Read the model definition and answer for the solid it produces. Units are mm, in the model's axes. Give positions to 0.01 mm unless a question says otherwise; leave off trailing zeros. Order: outer loops, then holes, each group sorted by start corner. A loop starts at its lowest first (then second) coordinate and runs counter-clockwise, first axis right, second up. Notation, with made-up numbers: (-5, 53) - (39, 53) arc R12 cw to (39, 59) - close; hole circle Ø6 at (17.25, -33.75). An arc over 180 degrees is marked (long way). Write each question's results on one line, items separated by ' | '. Start each with the question number.
Q1. Find the intervals of material crossed by line 1 along Z through (x, y) = (-101.5, 1); line 2 along Z through (x, y) = (92.5, 2.85); line 3 along Z through (x, y) = (72, 1.65), in increasing order. Write a range as from..to.
Q2. A flat-ended cylindrical pin translates along its axis: P1, Ø1, axis at y = 2.5, z = -94, coming from the +X side. Find the tip coordinate at first contact, or state that the pin passes through.
Q3. Find section A-A on x = 40. Give the vertices of the cut face in (y, z) (3 decimals), and give its area (3 significant figures).
Q4. Find section B-B on z = -66. Give the vertices of the cut face in (x, y) (3 decimals), and give its area (3 significant figures).
Q5. Find section C-C on y = 1.45. Count the separate pieces of the cut face and the enclosed holes in it, and give its area (3 significant figures).
Autodesk Inventor part; units mm, degrees
ref_plane "YZ Plane" through (0, 0, 0) normal (1, 0, 0) x (0, 1, 0)
ref_plane "XZ Plane" through (0, 0, 0) normal (0, 1, 0) x (-1, 0, 0)
ref_plane "XY Plane" through (0, 0, 0) normal (0, 0, 1) x (1, 0, 0)
sketch "Sketch1" plane through (0, 0, 0) normal (0, 1, 0) x (-1, 0, 0)
  line L0 (147.066, 381) -> (0, 381)
  line L1 (-147.066, 33.688) -> (-147.066, -381)
  line L2 (-147.066, -381) -> (147.066, -381)
  line L3 (147.066, -381) -> (147.066, 381)
  line L4 (147.066, 381) -> (-147.066, -381) construction
  line L5 (136.271, -185.928) -> (115.951, -185.928) construction
  line L6 (115.951, -185.928) -> (115.951, -231.648) construction
  line L7 (115.951, -231.648) -> (136.271, -231.648) construction
  line L8 (136.271, -231.648) -> (136.271, -185.928) construction
  line L9 (136.271, -185.928) -> (115.951, -231.648) construction
  line L10 (115.951, -185.928) -> (136.271, -231.648) construction
  circle A0 centre (126.111, -231.648) radius 3.556
  circle A1 centre (126.111, -185.928) radius 3.556
  circle A2 centre (126.111, -208.788) radius 3.556
  line L11 (0, 0) -> (147.066, 0) construction
  line L12 (136.271, 231.648) -> (115.951, 231.648) construction
  line L13 (115.951, 231.648) -> (115.951, 185.928) construction
  line L14 (115.951, 185.928) -> (136.271, 185.928) construction
  line L15 (136.271, 185.928) -> (136.271, 231.648) construction
  line L16 (136.271, 231.648) -> (115.951, 185.928) construction
  line L17 (115.951, 231.648) -> (136.271, 185.928) construction
  circle A3 centre (126.111, 231.648) radius 3.556
  circle A4 centre (126.111, 208.788) radius 3.556
  circle A5 centre (126.111, 185.928) radius 3.556
  line L18 (0, 381) -> (-147.066, 381)
  line L19 (-147.066, 381) -> (-147.066, 33.688)
  line L20 (0, 215.9) -> (-147.066, 215.9)
  line L21 (-147.066, 215.9) -> (-147.066, -215.9)
  line L22 (-147.066, -215.9) -> (0, -215.9)
  line L23 (0, -215.9) -> (0, 215.9)
  line L24 (0, 215.9) -> (-147.066, -215.9) construction
  line L25 (-147.066, 215.9) -> (0, -215.9) construction
  point P0 (-73.533, 0)
  dimension "d1" = 294.132
  dimension "d8" = 20.955
  dimension "d9" = 762
  dimension "d10" = 20.32
  dimension "d11" = 45.72
  dimension "d12" = 7.112
  dimension "d13" = 7.112
  dimension "d14" = 7.112
  dimension "d15" = 149.352
  dimension "d16" = 45.72
  dimension "d17" = 149.352
  dimension "d18" = 7.112
  dimension "d19" = 7.112
  dimension "d20" = 7.112
  dimension "d21" = 431.8
  dimension "d22" = 147.066
  dimension "d23" = 0
extrude "Extrusion1" add sketch "Sketch1" along normal blind 3.175 contours L3 L2 L1 L22 L23 L20 L19 L18 L0
sketch "Sketch2" plane through (0, 3.175, 0) normal (0, 1, 0) x (1, 0, 0)
  line L0 (-121.666, 364.3122) -> (-96.266, 364.3122) construction
  line L1 (-121.666, 359.8672) -> (-96.266, 359.8672)
  line L2 (-96.266, 368.7572) -> (-121.666, 368.7572)
  arc A0 (-121.666, 368.7572) -> (-121.666, 359.8672) centre (-121.666, 364.3122) ccw
  arc A1 (-96.266, 359.8672) -> (-96.266, 368.7572) centre (-96.266, 364.3122) ccw
  line L3 (147.066, 381) -> (-147.066, 381)
  line L4 (-70.866, 364.3122) -> (-45.466, 364.3122) construction
  line L5 (-70.866, 359.8672) -> (-45.466, 359.8672)
  line L6 (-45.466, 368.7572) -> (-70.866, 368.7572)
  arc A2 (-70.866, 368.7572) -> (-70.866, 359.8672) centre (-70.866, 364.3122) ccw
  arc A3 (-45.466, 359.8672) -> (-45.466, 368.7572) centre (-45.466, 364.3122) ccw
  line L7 (-20.066, 364.3122) -> (5.334, 364.3122) construction
  line L8 (-20.066, 359.8672) -> (5.334, 359.8672)
  line L9 (5.334, 368.7572) -> (-20.066, 368.7572)
  arc A4 (-20.066, 368.7572) -> (-20.066, 359.8672) centre (-20.066, 364.3122) ccw
  arc A5 (5.334, 359.8672) -> (5.334, 368.7572) centre (5.334, 364.3122) ccw
  line L10 (30.734, 364.3122) -> (56.134, 364.3122) construction
  line L11 (30.734, 359.8672) -> (56.134, 359.8672)
  line L12 (56.134, 368.7572) -> (30.734, 368.7572)
  arc A6 (30.734, 368.7572) -> (30.734, 359.8672) centre (30.734, 364.3122) ccw
  arc A7 (56.134, 359.8672) -> (56.134, 368.7572) centre (56.134, 364.3122) ccw
  line L13 (-147.066, 381) -> (-147.066, -381)
  line L14 (0, 0) -> (-147.066, 0) construction
  line L15 (-121.666, -364.3122) -> (-96.266, -364.3122) construction
  line L16 (-121.666, -359.8672) -> (-96.266, -359.8672)
  line L17 (-96.266, -368.7572) -> (-121.666, -368.7572)
  arc A8 (-121.666, -359.8672) -> (-121.666, -368.7572) centre (-121.666, -364.3122) ccw
  arc A9 (-96.266, -368.7572) -> (-96.266, -359.8672) centre (-96.266, -364.3122) ccw
  line L18 (-70.866, -364.3122) -> (-45.466, -364.3122) construction
  line L19 (-70.866, -359.8672) -> (-45.466, -359.8672)
  line L20 (-45.466, -368.7572) -> (-70.866, -368.7572)
  arc A10 (-70.866, -359.8672) -> (-70.866, -368.7572) centre (-70.866, -364.3122) ccw
  arc A11 (-45.466, -368.7572) -> (-45.466, -359.8672) centre (-45.466, -364.3122) ccw
  line L21 (-20.066, -364.3122) -> (5.334, -364.3122) construction
  line L22 (-20.066, -359.8672) -> (5.334, -359.8672)
  line L23 (5.334, -368.7572) -> (-20.066, -368.7572)
  arc A12 (-20.066, -359.8672) -> (-20.066, -368.7572) centre (-20.066, -364.3122) ccw
  arc A13 (5.334, -368.7572) -> (5.334, -359.8672) centre (5.334, -364.3122) ccw
  line L24 (30.734, -364.3122) -> (56.134, -364.3122) construction
  line L25 (30.734, -359.8672) -> (56.134, -359.8672)
  line L26 (56.134, -368.7572) -> (30.734, -368.7572)
  arc A14 (30.734, -359.8672) -> (30.734, -368.7572) centre (30.734, -364.3122) ccw
  arc A15 (56.134, -368.7572) -> (56.134, -359.8672) centre (56.134, -364.3122) ccw
  circle A16 centre (-108.966, 337.185) radius 4.7625
  circle A17 centre (108.966, 337.185) radius 4.7625
  line L27 (147.066, 215.9) -> (147.066, 381)
  circle A18 centre (-108.966, -337.185) radius 4.7625
  circle A19 centre (108.966, -337.185) radius 4.7625
  line L28 (78.7859, 364.3122) -> (104.1859, 364.3122) construction
  line L29 (78.7859, 359.8672) -> (104.1859, 359.8672)
  line L30 (104.1859, 368.7572) -> (78.7859, 368.7572)
  arc A20 (78.7859, 368.7572) -> (78.7859, 359.8672) centre (78.7859, 364.3122) ccw
  arc A21 (104.1859, 359.8672) -> (104.1859, 368.7572) centre (104.1859, 364.3122) ccw
  line L31 (78.7859, -364.3122) -> (104.1859, -364.3122) construction
  line L32 (78.7859, -359.8672) -> (104.1859, -359.8672)
  line L33 (104.1859, -368.7572) -> (78.7859, -368.7572)
  arc A22 (78.7859, -359.8672) -> (78.7859, -368.7572) centre (78.7859, -364.3122) ccw
  arc A23 (104.1859, -368.7572) -> (104.1859, -359.8672) centre (104.1859, -364.3122) ccw
  point P0 (-108.966, 364.3122)
  point P1 (-58.166, 364.3122)
  point P2 (-7.366, 364.3122)
  point P3 (43.434, 364.3122)
  point P4 (-108.966, -364.3122)
  point P5 (-58.166, -364.3122)
  point P6 (-7.366, -364.3122)
  point P7 (43.434, -364.3122)
  point P8 (91.4859, 364.3122)
  point P9 (91.4859, -364.3122)
  dimension "d24" = 8.89
  dimension "d25" = 16.6878
  dimension "d26" = 25.4
  dimension "d27" = 25.4
  dimension "d28" = 8.89
  dimension "d29" = 25.4
  dimension "d30" = 8.89
  dimension "d31" = 25.4
  dimension "d32" = 8.89
  dimension "d33" = 25.4
  dimension "d34" = 25.4
  dimension "d35" = 25.4
  dimension "d36" = 25.4
  dimension "d42" = 9.525
  dimension "d43" = 43.815
  dimension "d44" = 38.1
  dimension "d45" = 9.525
  dimension "d46" = 43.815
  dimension "d47" = 38.1
  dimension "d48" = 25.4
  dimension "d49" = 4.445
extrude "Extrusion2" cut sketch "Sketch2" against normal blind 3.175
equation "\"d12\" = d13"
equation "\"d14\" = d13"
equation "\"d16\" = d11"
equation "\"d17\" = d15"
equation "\"d18\" = d13"
equation "\"d19\" = d13"
equation "\"d20\" = d13"
equation "\"d27\" = d26"
equation "\"d29\" = d26"
equation "\"d31\" = d26"
equation "\"d33\" = d36"
equation "\"d34\" = d36"
equation "\"d35\" = d36"
equation "\"d45\" = d42"
equation "\"d46\" = d43"
equation "\"d47\" = d44"
equation "\"d48\" = d31"
equation "\"d49\" = 0.5 * d32"
properties part number "lid"
Working result:
1) line 1: -381..-368.76, -359.87..359.87, 368.76..381 | line 2: -381..-368.76, -359.87..-215.9, 215.9..359.87, 368.76..381 | line 3: -381..-215.9, 215.9..381
2) P1: x = 0
3) outline: (0, -381) - (3.175, -381) - (3.175, -368.757) - (0, -368.757) - close; (0, -359.867) - (3.175, -359.867) - (3.175, -215.9) - (0, -215.9) - close; (0, 215.9) - (3.175, 215.9) - (3.175, 359.867) - (0, 359.867) - close; (0, 368.757) - (3.175, 368.757) - (3.175, 381) - (0, 381) - close | area: 992 mm²
4) outline: (-147.066, 0) - (0, 0) - (0, 3.175) - (-147.066, 3.175) - close | area: 467 mm²
5) separate pieces: 1 | enclosed holes: 20 | area: 157,000 mm²
